```python
from build123d import *

# Parameters (mm, degrees)
F1_DEPTH = 950
F2_R     = 6.25
F3_DEPTH = 100.001
F4_R     = 6.25
F5_DEPTH = 100.001


with BuildPart() as f1:
    # F0 (on Front) → F1 (new body, symmetric)
    with BuildSketch(Plane.XZ):
        with BuildLine():
            Line((-40, -50), (40, -50))
            ThreePointArc((40, -50), (47.071068, -47.071068), (50, -40))
            Line((50, -40), (50, 40))
            ThreePointArc((50, 40), (47.071068, 47.071068), (40, 50))
            Line((40, 50), (-40, 50))
            ThreePointArc((-40, 50), (-47.071068, 47.071068), (-50, 40))
            Line((-50, 40), (-50, -40))
            ThreePointArc((-50, -40), (-47.071068, -47.071068), (-40, -50))
        make_face()
        with BuildLine():
            ThreePointArc((40, 45), (43.535534, 43.535534), (45, 40))
            Line((45, 40), (45, -40))
            ThreePointArc((45, -40), (43.535534, -43.535534), (40, -45))
            Line((40, -45), (-40, -45))
            ThreePointArc((-40, -45), (-43.535534, -43.535534), (-45, -40))
            Line((-45, -40), (-45, 40))
            ThreePointArc((-45, 40), (-43.535534, 43.535534), (-40, 45))
            Line((-40, 45), (40, 45))
        make_face(mode=Mode.SUBTRACT)
    extrude(amount=F1_DEPTH, both=True)

    # F2 (on face) → F3 (cut, through all)
    with BuildSketch(Plane.YZ.offset(50)):
        with Locations((-907.5, 25)):
            Circle(F2_R)
        with Locations((-842.5, 25)):
            Circle(F2_R)
        with Locations((-842.5, -25)):
            Circle(F2_R)
        with Locations((-907.5, -25)):
            Circle(F2_R)
    extrude(amount=-F3_DEPTH, mode=Mode.SUBTRACT)

    # F4 (on face) → F5 (cut, through all)
    with BuildSketch(Plane.YZ.offset(50)):
        with Locations((870, 31)):
            Circle(F4_R)
        with Locations((924.378467, 5.642904)):
            Circle(F4_R)
        with Locations((907.473737, -30.609407)):
            Circle(F4_R)
        with Locations((853.09527, -5.252311)):
            Circle(F4_R)
    extrude(amount=-F5_DEPTH, mode=Mode.SUBTRACT)


solid = f1.part
```
Work out the finished part from the listing and answer in its coordinate system (mm). A direction names the side the tool comes from. Give positions to 0.01 mm unless a question says otherwise; leave off trailing zeros. Order: outer loops, then holes, each group sorted by start corner. A loop starts at its lowest first (then second) coordinate and runs counter-clockwise, first axis right, second up. Notation, with made-up numbers: (10.5, 84.25) - (23.5, 84.25) arc R9 ccw to (23.5, 101.25) - close; hole circle Ø9 at (45.5, -19.75). An arc over 180 degrees is marked (long way). One line per item, written item: value. Start each with the question number.
1. Section A-A, the plane x = 8.5 is taken. Write down the section's boundary in (y, z).
2. For a pull along X with two mould halves and no side action, classify faces 1 (the face through (-50, -13, 1)), 2 (the face through (-4, -950, -48)), 3 (the face through (45, -13, 1)) as released by +X, released by -X, zero draft, split by the parting line, or undercut.
3. This flat-tipped pin is pushed along its axis until it touches: pin 1 Ø7.5 at (y, z) = (853.1, -5.25) entering from +X. Where does it stop, or does it pass through?
4. Consider line 1 (Z direction, x = 35, y = 432); line 2 (Z direction, x = 47.2, y = -842.5). Determine where each line is inside the solid, lowest interval first.
5. Which of the six approach directions +Z, -Z, +X, -X, +Y, -Y give full straight-line access (tool end or side, diameter ignored) to faces 4 (the face through (-45, -13, -1)), 5 (the face through (-4, 950, -48))?
6. Section B-B, the plane y = -102.5 is taken. Write down the section's boundary in (x, z), then the cut area to 3 significant figures.
Filled sheet:
1. outline: (-950, -50) - (950, -50) - (950, -45) - (-950, -45) - close; (-950, 45) - (950, 45) - (950, 50) - (-950, 50) - close
2. face 1: released by -X
2. face 2: zero draft
2. face 3: undercut
3. pin 1: through
4. line 1: -50 to -45, 45 to 50
4. line 2: -46.94 to -31.25, -18.75 to 18.75, 31.25 to 46.94
5. face 4: +Y, -Y
5. face 5: +Z, -Z, +X, -X, +Y
6. outline: (-50, -40) arc R10 ccw to (-40, -50) - (40, -50) arc R10 ccw to (50, -40) - (50, 40) arc R10 ccw to (40, 50) - (-40, 50) arc R10 ccw to (-50, 40) - close; hole (-45, -40) arc R5 ccw to (-40, -45) - (40, -45) arc R5 ccw to (45, -40) - (45, 40) arc R5 ccw to (40, 45) - (-40, 45) arc R5 ccw to (-45, 40) - close
6. area: 1,840 mm²
